```python
from build123d import *

# Parameters (mm, degrees)
SKETCH_1_R      = 1.75
SKETCH_1_R_2    = 3.5
SKETCH_1_R_3    = 8
SKETCH_1_R_4    = 1
SKETCH_1_W      = 65
SKETCH_1_H      = 16.85
EXTRUDE_1_DEPTH = 1.6


with BuildPart() as part:
    # 草图1 → 凸台-拉伸1 (new body)
    with BuildSketch(Plane.XY):
        with BuildLine():
            Line((-57, 33.073154828), (57, 33.073154828))
            ThreePointArc((57, 33.073154828), (59.121320344, 32.194475172), (60, 30.073154828))
            Line((60, 30.073154828), (60, -22.926845172))
            ThreePointArc((60, -22.926845172), (59.121320344, -25.048165515), (57, -25.926845172))
            Line((57, -25.926845172), (-57, -25.926845172))
            ThreePointArc((-57, -25.926845172), (-59.121320344, -25.048165515), (-60, -22.926845172))
            Line((-60, -22.926845172), (-60, 30.073154828))
            ThreePointArc((-60, 30.073154828), (-59.121320344, 32.194475172), (-57, 33.073154828))
        make_face()
        with Locations((-55, -20.926845172)):
            Circle(SKETCH_1_R, mode=Mode.SUBTRACT)
        with Locations((55, -20.926845172)):
            Circle(SKETCH_1_R, mode=Mode.SUBTRACT)
        with Locations((55, 28.073154828)):
            Circle(SKETCH_1_R, mode=Mode.SUBTRACT)
        with Locations((-55, 28.073154828)):
            Circle(SKETCH_1_R, mode=Mode.SUBTRACT)
        with Locations((26.721118862, -13.682497654)):
            Circle(SKETCH_1_R_2, mode=Mode.SUBTRACT)
        with Locations((-18.798880758, -13.312497654)):
            Circle(SKETCH_1_R_3, mode=Mode.SUBTRACT)
        with Locations((8.251119242, -12.222497654)):
            Circle(SKETCH_1_R_4, mode=Mode.SUBTRACT)
        with Locations((0.097411242, 12.102502346)):
            Rectangle(SKETCH_1_W, SKETCH_1_H, mode=Mode.SUBTRACT)
    extrude(amount=EXTRUDE_1_DEPTH)


solid = part.part
```
Verification items for the finished model (mm, model axes). Round coordinates to 2 decimals unless told otherwise and drop trailing zeros. Loops run counter-clockwise (first coordinate to the right, second up) from the corner with the lowest first, then second, coordinate; pieces in that order, holes last. Notation, with made-up numbers: (77, 40.5) -> (82, 40.5) arc R21 cw to (82, 60.5) -> close; hole circle Ø7 at (87, 30.25). An arc over 180 degrees is marked (long way). Answer as a JSON object with one key per item and string values.
Q1. Section check C-C (x = -31). Record the boundary of the cut face in (y, z).
Data:
{"outline": "(-25.93, 0) -> (3.68, 0) -> (3.68, 1.6) -> (-25.93, 1.6) -> close; (20.53, 0) -> (33.07, 0) -> (33.07, 1.6) -> (20.53, 1.6) -> close"}
Q2. Scan lines: line 1 (Y direction, x = 55, z = 0.9); line 2 (X direction, y = 16, z = 1.1); line 3 (Y direction, x = -25, z = 1.2). Record each from-to range of solid material in increasing order. Write a range as from..to.
Data:
{"line 1": "y = -25.93..-22.68, -19.18..26.32, 29.82..33.07", "line 2": "x = -60..-32.4, 32.6..60", "line 3": "y = -25.93..-18.37, -8.26..3.68, 20.53..33.07"}
Q3. Section check B-B (x = -55). Record the boundary of the cut face in (y, z).
Data:
{"outline": "(-25.93, 0) -> (-22.68, 0) -> (-22.68, 1.6) -> (-25.93, 1.6) -> close; (-19.18, 0) -> (26.32, 0) -> (26.32, 1.6) -> (-19.18, 1.6) -> close; (29.82, 0) -> (33.07, 0) -> (33.07, 1.6) -> (29.82, 1.6) -> close"}
Q4. Section check D-D (z = 1.05). State how many separate pieces and enclosed holes the cut face has, then the cut area to 3 significant figures.
Data:
{"separate pieces": "1", "enclosed holes": "8", "area": "5,700 mm2"}
Q5. Section check A-A (y = 9). Record the boundary of the cut face in (x, z).
Data:
{"outline": "(-60, 0) -> (-32.4, 0) -> (-32.4, 1.6) -> (-60, 1.6) -> close; (32.6, 0) -> (60, 0) -> (60, 1.6) -> (32.6, 1.6) -> close"}
Q6. Draft check along X on faces 1 (the cylindrical face through (56.67, -20.4, 0.79)), 2 (the cylindrical face through (-59.145, 32.171, 0.789)), 3 (the flat face through (1, -3, 0)). Enter one of: pulls with the +X half, pulls with the -X half, needs draft (parallel to the pull), parting line crosses it, or undercut.
Data:
{"face 1": "undercut", "face 2": "pulls with the -X half", "face 3": "needs draft"}
